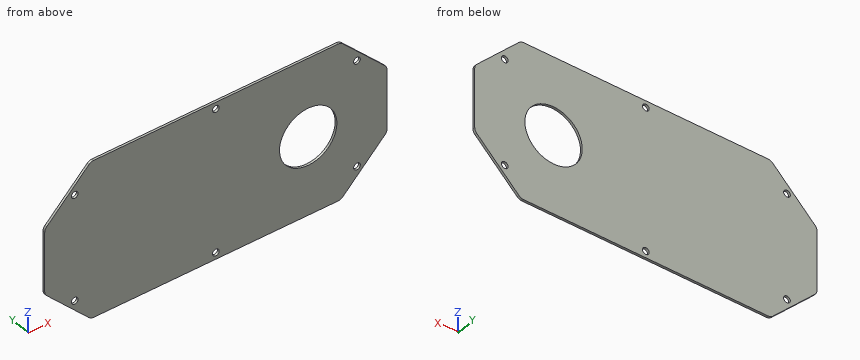
from build123d import *

# Parameters (mm, degrees)
SM_BASE_FLANGE_1_DEPTH = 1
SKETCH_2_R             = 1.5
CUT_EXTRUDE_1_DEPTH    = 10
FILLET_1_R             = 3
SKETCH_3_R             = 12.75
CUT_EXTRUDE_2_DEPTH    = 10


# Sheet-metal steps are written as plain solids
with BuildPart() as part:
    # Sketch 1 → Базовая кромка1 (new body)
    with BuildSketch(Plane(origin=(0, 0, 0), x_dir=(1, 0, 0), z_dir=(0, 1, 0))):
        Polygon((-96.502525317, -35), (14.497474683, -35), (35, -14.497474683), (35, 14.497474683), (14.497474683, 35), (-96.502525317, 35), (-117.005525317, 14.497), (-117.005525317, 0), (-117.005525317, -14.497), align=None)
    extrude(amount=-SM_BASE_FLANGE_1_DEPTH)

    # Эскиз2 → Вырез-Вытянуть1 (cut)
    with BuildSketch(Plane(origin=(0, 0, 0), x_dir=(1, 0, 0), z_dir=(0, 1, 0))):
        with Locations(Location((-103.671600061, 23.588284569, 0), (0, 0, 270))):
            Circle(SKETCH_2_R)
        with Locations(Location((-41.002525317, 32, 0), (0, 0, 270))):
            Circle(SKETCH_2_R)
        with Locations(Location((21.666312086, 23.58852191, 0), (0, 0, 270))):
            Circle(SKETCH_2_R)
        with Locations(Location((21.666312086, -23.58852191, 0), (0, 0, 270))):
            Circle(SKETCH_2_R)
        with Locations(Location((-103.671600061, -23.588284569, 0), (0, 0, 270))):
            Circle(SKETCH_2_R)
        with Locations(Location((-41.002525317, -32, 0), (0, 0, 270))):
            Circle(SKETCH_2_R)
    extrude(amount=-CUT_EXTRUDE_1_DEPTH, mode=Mode.SUBTRACT)

    # Скругление1
    fillet_1_edges = [part.edges().sort_by_distance(p)[0] for p in [
        (-117.005525317, -0.5, 14.497),
        (-117.005525317, -0.5, -14.497),
        (-96.502525317, -0.5, -35),
        (14.497474683, -0.5, -35),
        (35, -0.5, -14.497474683),
        (35, -0.5, 14.497474683),
        (14.497474683, -0.5, 35),
        (-96.502525317, -0.5, 35),
    ]]
    fillet(fillet_1_edges, radius=FILLET_1_R)

    # Эскиз3 → Вырез-Вытянуть2 (cut)
    with BuildSketch(Plane.XZ.offset(1)):
        with Locations(Location((0, 0, 0), (0, 0, 270))):
            Circle(SKETCH_3_R)
    extrude(amount=-CUT_EXTRUDE_2_DEPTH, mode=Mode.SUBTRACT)


solid = part.part
CAD build for the part. Positions are in the model's coordinates, mm. Give positions to 0.01 mm unless a question says otherwise; leave off trailing zeros. Write each loop counter-clockwise with the first axis right and the second up, starting at its lowest first coordinate (ties: lowest second). Pieces come first, ordered by that corner, then holes. Notation, with made-up numbers: (42, -18.75) -> (68, -18.75) arc R29 cw to (68, 7.25) -> close; hole circle Ø9 at (38.25, -36.5). An arc over 180 degrees is marked (long way). Return JSON: item names as keys, results as strings.
Item 1: Band-saw the part on C-C (y = -0.3). List the corners of the cut face in (x, z), then the cut area to 4 significant figures.
Answer below:
{"outline": "(-117.01, -13.25) arc R3 ccw to (-116.13, -15.38) -> (-97.38, -34.12) arc R3 ccw to (-95.26, -35) -> (13.25, -35) arc R3 ccw to (15.38, -34.12) -> (34.12, -15.38) arc R3 ccw to (35, -13.25) -> (35, 13.25) arc R3 ccw to (34.12, 15.38) -> (15.38, 34.12) arc R3 ccw to (13.25, 35) -> (-95.26, 35) arc R3 ccw to (-97.38, 34.12) -> (-116.13, 15.38) arc R3 ccw to (-117.01, 13.25) -> close; hole circle Ø3 at (-103.67, -23.59); hole circle Ø3 at (-103.67, 23.59); hole circle Ø3 at (-41, -32); hole circle Ø3 at (-41, 32); hole circle Ø25.5 at (0, 0); hole circle Ø3 at (21.67, -23.59); hole circle Ø3 at (21.67, 23.59)", "area": "9,245 mm2"}
Item 2: Band-saw the part on A-A (z = 0). List the corners of the cut face in (x, y).
Answer below:
{"outline": "(-117.01, -1) -> (-12.75, -1) -> (-12.75, 0) -> (-117.01, 0) -> close; (12.75, -1) -> (35, -1) -> (35, 0) -> (12.75, 0) -> close"}
Item 3: Band-saw the part on D-D (z = 19.5). List the corners of the cut face in (x, y), then the cut area to 3 significant figures.
Answer below:
{"outline": "(-112, -1) -> (30, -1) -> (30, 0) -> (-112, 0) -> close", "area": "142 mm2"}
Item 4: Drill centre lines: probe 1 along X at (y, z) = (-0.45, 0); probe 2 along X at (y, z) = (-0.65, -24); probe 3 along Z at (x, y) = (21.5, -0.1). Where is each one in solid material? Low to high.
Answer below:
{"probe 1": "x = -117.01 to -12.75, 12.75 to 35", "probe 2": "x = -107.5 to -105.11, -102.23 to 20.22, 23.11 to 25.5", "probe 3": "z = -28 to -25.08, -22.1 to 22.1, 25.08 to 28"}
Item 5: Band-saw the part on B-B (x = 0). List the corners of the cut face in (y, z), then the cut area to 3 significant figures.
Answer below:
{"outline": "(-1, -35) -> (0, -35) -> (0, -12.75) -> (-1, -12.75) -> close; (-1, 12.75) -> (0, 12.75) -> (0, 35) -> (-1, 35) -> close", "area": "44.5 mm2"}
Item 6: Drop a flat-ended pin along its axis: pin 1 (10 mm diameter, centred on x = 7, z = -2, fed in from -Y). Give the stop position or say it passes through.
Answer below:
{"pin 1": "passes through"}
